The figure shows three views and two pictorial views of one solid part (mm, origin at its lowest corner). Answer the questions. Round coordinates to 2 decimals unless told otherwise and drop trailing zeros. Order: outer loops, then holes, each group sorted by start corner. A loop starts at its lowest first (then second) coordinate and runs counter-clockwise, first axis right, second up. Notation, with made-up numbers: M 48,64 L 64,64 A13 ccw 64,84 Z; hole C 60.5,36.5 d1. An arc over 180 degrees is marked long. Return JSON: item names as keys, results as strings.
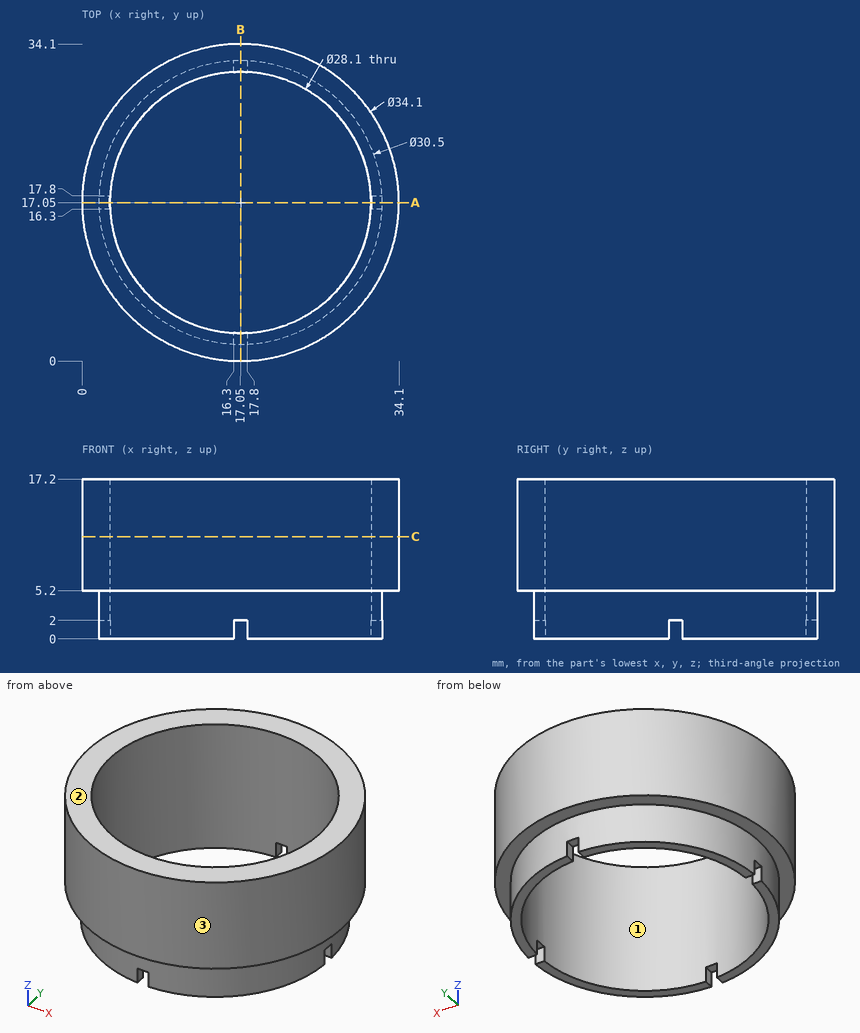
Item 1: Find section A-A (y = 17.05). Determine the outline of the cut face in (x, z).
Output:
{"outline": "M 0,5.2 L 1.8,5.2 L 1.8,2 L 3,2 L 3,17.2 L 0,17.2 Z; M 31.1,2 L 32.3,2 L 32.3,5.2 L 34.1,5.2 L 34.1,17.2 L 31.1,17.2 Z"}
Item 2: The mould has two halves that part along Y. Classify the marked faces 1, 2 and 3: pulls with the +Y half, pulls with the -Y half, needs draft (parallel to the pull), parting line crosses it, or undercut.
Output:
{"face 1": "undercut", "face 2": "needs draft", "face 3": "parting line crosses it"}
Item 3: Consider line 1 along Y through (x, z) = (17.05, 9); line 2 along Y through (x, z) = (17.05, 3.5). Determine where each line is inside the solid, lowest interval first. Write a range as [from, to].
Output:
{"line 1": "y = [0, 3], [31.1, 34.1]", "line 2": "y = [1.8, 3], [31.1, 32.3]"}
Item 4: Find section C-C (z = 11). Determine the outline of the cut face in (x, y).
Output:
{"outline": "C 17.05,17.05 d34.1; hole C 17.05,17.05 d28.1"}
Item 5: Each of these flat-tipped pins is pushed along its axis until it touches: pin 1 (1.3 mm diameter, centred on x = 17, y = 32, fed in from -Z); pin 2 (1 mm diameter, centred on x = 2.5, z = 1, fed in from -Y); pin 3 (1 mm diameter, centred on x = 22.5, z = 12, fed in from -Y); pin 4 (6 mm diameter, centred on x = 23.5, y = 24.5, fed in from +Z). Where does it stop, or does it pass through?
Output:
{"pin 1": "stops at z = 2", "pin 2": "stops at y = 11.12", "pin 3": "stops at y = 0.73", "pin 4": "passes through"}
